Here's how the part is built. I have some questions about the finished solid (model axes, mm). A direction names the side the tool comes from. Coordinates: 2 decimals unless noted, no trailing zeros. Loops run counter-clockwise (first coordinate to the right, second up) from the corner with the lowest first, then second, coordinate; pieces in that order, holes last. Notation, with made-up numbers: M 47,52.25 L 96,52.25 A19 cw 96,58.25 Z; hole C 31,-32 d1. An arc over 180 degrees is marked long. Use CSV: the item, a comma, the result in double quotes. Start each with the question number.
Q1. Please list where these lines run through material, in increasing order: probe 1 along X at (y, z) = (18, 60.5); probe 2 along Y at (x, z) = (19.45, 470); probe 3 along Y at (x, z) = (17.5, 187). Write a range as [from, to].
Q2. Which directions (+Z, -Z, +X, -X, +Y, -Y) give clear straight access to the entire face, cutting with the end or side of a thin tool? Please do faces 5 (the flat face through (18, 20, 246)), 6 (the flat face through (1.8, 21.6, 500)).
Q3. If we section it at A-A (x = 9.25): Please give me the cut outline in (y, z), and give its area (3 significant figures).
Q4. If we section it at C-C (y = 17.5): Please give me the cut outline in (x, z), and give its area (3 significant figures).
Q5. If we mould it in two halves opening along Y, with no side actions, what happens to faces 1 (the flat face through (10, 40, 246)), 2 (the flat face through (1.8, 21.6, 0)), 3 (the flat face through (10, 38, 246)), 4 (the flat face through (10, 0, 246))? For each: +Y half, -Y half, draft (parallel to the pull), parting line (faces both ways), or undercut.
Q6. If we section it at B-B (z = 56): Please give me the cut outline in (x, y).
from build123d import *

# Parameters (mm, degrees)
ESBO_O1_W                = 20
ESBO_O1_H                = 40
ESBO_O1_W_2              = 16
ESBO_O1_H_2              = 36
RESSALTO_EXTRUS_O1_DEPTH = 500
ESBO_O2_R                = 1.75
CORTE_EXTRUS_O1_DEPTH    = 2
CORTE_EXTRUS_O2_START    = -2
ESBO_O5_R                = 1.75
CORTE_EXTRUS_O2_DEPTH    = 2


with BuildPart() as part:
    # Esboço1 → Ressalto-extrusão1 (new body)
    with BuildSketch(Plane.XY):
        with Locations((10, 20)):
            Rectangle(ESBO_O1_W, ESBO_O1_H)
        with Locations((10, 20)):
            Rectangle(ESBO_O1_W_2, ESBO_O1_H_2, mode=Mode.SUBTRACT)
    extrude(amount=RESSALTO_EXTRUS_O1_DEPTH)

    # Esboço2 → Corte-extrusão1 (cut)
    with BuildSketch(Plane.ZY):
        with Locations((15, 10)):
            Circle(ESBO_O2_R)
        with Locations((30, 10)):
            Circle(ESBO_O2_R)
        with Locations(Location((485, 10, 0), (0, 0, 180))):
            Circle(ESBO_O2_R)
        with Locations(Location((470, 10, 0), (0, 0, 180))):
            Circle(ESBO_O2_R)
    extrude(amount=-CORTE_EXTRUS_O1_DEPTH, mode=Mode.SUBTRACT)

    # Esboço5 → Corte-extrusão2 (cut)
    with BuildSketch(Plane(origin=(20, 0, 0), x_dir=(0, 0, -1), z_dir=(1, 0, 0)).offset(CORTE_EXTRUS_O2_START)):
        with Locations(Location((-15, 10, 0), (0, 0, 180))):
            Circle(ESBO_O5_R)
        with Locations(Location((-30, 10, 0), (0, 0, 180))):
            Circle(ESBO_O5_R)
        with Locations((-485, 10)):
            Circle(ESBO_O5_R)
        with Locations((-470, 10)):
            Circle(ESBO_O5_R)
    extrude(amount=CORTE_EXTRUS_O2_DEPTH, mode=Mode.SUBTRACT)


solid = part.part
Results below:
1,probe 1,"[0, 2], [18, 20]"
1,probe 2,"[0, 8.25], [11.75, 40]"
1,probe 3,"[0, 2], [38, 40]"
2,face 5,"+Z, -Z"
2,face 6,"+Z, +X, -X, +Y, -Y"
3,outline,"M 0,0 L 2,0 L 2,500 L 0,500 Z; M 38,0 L 40,0 L 40,500 L 38,500 Z"
3,area,"2,000 mm^2"
4,outline,"M 0,0 L 2,0 L 2,500 L 0,500 Z; M 18,0 L 20,0 L 20,500 L 18,500 Z"
4,area,"2,000 mm^2"
5,face 1,"+Y half"
5,face 2,"draft"
5,face 3,"undercut"
5,face 4,"-Y half"
6,outline,"M 0,0 L 20,0 L 20,40 L 0,40 Z; hole M 2,2 L 18,2 L 18,38 L 2,38 Z"
